from build123d import *

# Parameters (mm, degrees)
F0_W      = 57
F0_H      = 57
F1_DEPTH  = 49
F2_R      = 2
F3_R      = 2.55
F4_DEPTH  = 49.001
F5_R      = 2.55
F6_DEPTH  = 44
F7_R      = 3
F8_R      = 10
F9_DEPTH  = 2
F10_R     = 4
F11_DEPTH = 25
F12_R     = 19
F12_R_2   = 10
F13_DEPTH = 1.5


with BuildPart() as f1:
    # F0 (on Top) → F1 (new body)
    with BuildSketch(Plane.XY):
        Rectangle(F0_W, F0_H)
    extrude(amount=F1_DEPTH)

    # F2
    f2_edges = [f1.edges().sort_by_distance(p)[0] for p in [
        (-28.5, -28.5, 24.5),
        (28.5, -28.5, 24.5),
        (28.5, 28.5, 24.5),
        (-28.5, 28.5, 24.5),
    ]]
    fillet(f2_edges, radius=F2_R)

    # F3 (on face) → F4 (cut, through all)
    with BuildSketch(Plane(origin=(0, 0, 0), x_dir=(1, 0, 0), z_dir=(0, 0, -1))):
        with Locations((-23.5, -23.5)):
            Circle(F3_R)
        with Locations((-23.5, 23.5)):
            Circle(F3_R)
        with Locations((23.5, 23.5)):
            Circle(F3_R)
        with Locations((23.5, -23.5)):
            Circle(F3_R)
    extrude(amount=-F4_DEPTH, mode=Mode.SUBTRACT)

    # F5 (on face) → F6 (cut)
    with BuildSketch(Plane(origin=(0, 0, 0), x_dir=(1, 0, 0), z_dir=(0, 0, -1))):
        with BuildLine():
            Line((-26.5, -28.5), (-18.5, -28.5))
            Line((-18.5, -28.5), (-18.5, -18.5))
            Line((-18.5, -18.5), (-28.5, -18.5))
            Line((-28.5, -18.5), (-28.5, -26.5))
            ThreePointArc((-28.5, -26.5), (-27.9142135624, -27.9142135624), (-26.5, -28.5))
        make_face()
        with Locations((-23.5, -23.5)):
            Circle(F5_R, mode=Mode.SUBTRACT)
        with BuildLine():
            Line((28.5, -26.5), (28.5, -18.5))
            Line((28.5, -18.5), (18.5, -18.5))
            Line((18.5, -18.5), (18.5, -28.5))
            Line((18.5, -28.5), (26.5, -28.5))
            ThreePointArc((26.5, -28.5), (27.9142135624, -27.9142135624), (28.5, -26.5))
        make_face()
        with Locations((23.5, -23.5)):
            Circle(F5_R, mode=Mode.SUBTRACT)
        with BuildLine():
            Line((18.5, 18.5), (28.5, 18.5))
            Line((28.5, 18.5), (28.5, 26.5))
            ThreePointArc((28.5, 26.5), (27.9142135624, 27.9142135624), (26.5, 28.5))
            Line((26.5, 28.5), (18.5, 28.5))
            Line((18.5, 28.5), (18.5, 18.5))
        make_face()
        with Locations((23.5, 23.5)):
            Circle(F5_R, mode=Mode.SUBTRACT)
        with BuildLine():
            Line((-18.5, 18.5), (-18.5, 28.5))
            Line((-18.5, 28.5), (-26.5, 28.5))
            ThreePointArc((-26.5, 28.5), (-27.9142135624, 27.9142135624), (-28.5, 26.5))
            Line((-28.5, 26.5), (-28.5, 18.5))
            Line((-28.5, 18.5), (-18.5, 18.5))
        make_face()
        with Locations((-23.5, 23.5)):
            Circle(F5_R, mode=Mode.SUBTRACT)
    extrude(amount=-F6_DEPTH, mode=Mode.SUBTRACT)

    # F7
    f7_edges = [f1.edges().sort_by_distance(p)[0] for p in [
        (-18.5, -18.5, 22),
        (-18.5, -28.5, 22),
        (-28.5, -18.5, 22),
        (-28.5, 18.5, 22),
        (-18.5, 28.5, 22),
        (18.5, -28.5, 22),
        (28.5, -18.5, 22),
        (-18.5, 18.5, 22),
        (28.5, 18.5, 22),
        (18.5, 28.5, 22),
        (18.5, 18.5, 22),
        (18.5, -18.5, 22),
    ]]
    fillet(f7_edges, radius=F7_R)

    # F8 (on face) → F9 (cut)
    with BuildSketch(Plane.XY.offset(49)):
        Circle(F8_R)
    extrude(amount=-F9_DEPTH, mode=Mode.SUBTRACT)

    # F10 (on face) → F11 (cut)
    with BuildSketch(Plane.XY.offset(47)):
        Circle(F10_R)
    extrude(amount=-F11_DEPTH, mode=Mode.SUBTRACT)

    # F12 (on face) → F13 (join)
    with BuildSketch(Plane.XY.offset(49)):
        Circle(F12_R)
        Circle(F12_R_2, mode=Mode.SUBTRACT)
    extrude(amount=F13_DEPTH)


solid = f1.part
Read the model definition and answer for the solid it produces. Units are mm, in the model's axes. A direction names the side the tool comes from. Coordinates: 2 decimals unless noted, no trailing zeros. Order: outer loops, then holes, each group sorted by start corner. A loop starts at its lowest first (then second) coordinate and runs counter-clockwise, first axis right, second up. Notation, with made-up numbers: M 35.25,53.5 L 75.25,53.5 A32 cw 75.25,89.5 Z; hole C 42,31.5 d3. An arc over 180 degrees is marked long. Put each result on its own line as item: value. Start each with the question number.
Item 1: For faces 4 (the face through (27.64, -17.6, 22.31)), 5 (the face through (-23.54, 26.24, 44)), 6 (the face through (8, -8, 50.5)), 7 (the face through (24, 18.5, 22)), 8 (the face through (-23.5, -26.4, 44)), determine the directions among +Z, -Z, +X, -X, +Y, -Y from which every point of the face is accessible in a straight line to the end or side of a thin tool.
Item 2: Section A-A, the plane y = -23.5 is taken. Determine the outline of the cut face in (x, z), plus the area to 3 significant figures.
Item 3: Section B-B, the plane z = 30.5 is taken. Determine the outline of the cut face in (x, y).
Item 4: The mould has two halves that part along Y. Classify faces 1 (the face through (-25.4, -25.2, 46.5)), 2 (the face through (26.2, 23.4, 44)), 3 (the face through (27.93, 27.9, 46.54)): +Y half, -Y half, draft (parallel to the pull), parting line (faces both ways), or undercut.
Item 5: Section D-D, the plane y = 0 is taken. Determine the outline of the cut face in (x, z), plus the area to 3 significant figures.
Item 6: Consider probe 1 along X at (y, z) = (23.5, 46.95); probe 2 along Z at (x, y) = (4, 0.5). Determine where each line is inside the solid, lowest interval first. Write a range as [from, to].
Item 7: Given pin 1 Ø2 at (x, z) = (24.5, 31.5) entering from +Y; pin 2 Ø6 at (x, y) = (-9.5, 3) entering from -Z; pin 3 Ø2.5 at (x, y) = (0.5, -1.5) entering from +Z; pin 4 Ø4.5 at (x, z) = (24, 14.5) entering from -Y, each flat-ended and moving along its own axis, determine where each tip first touches the part or whether it passes through.
Computed:
1. face 4: -Z, +X, -Y
1. face 5: -Z, -X, +Y
1. face 6: +Z, +X, -X, +Y, -Y
1. face 7: -Z, +X, +Y
1. face 8: -Z, -X, -Y
2. outline: M -28.5,44 L -26.05,44 L -26.05,49 L -28.5,49 Z; M -20.95,44 L -18.5,44 L -18.5,0 L 18.5,0 L 18.5,44 L 20.95,44 L 20.95,49 L -20.95,49 Z; M 26.05,44 L 28.5,44 L 28.5,49 L 26.05,49 Z
2. area: 1,860 mm2
3. outline: M -28.5,-15.5 A3 ccw -25.5,-18.5 L -21.5,-18.5 A3 cw -18.5,-21.5 L -18.5,-25.5 A3 ccw -15.5,-28.5 L 15.5,-28.5 A3 ccw 18.5,-25.5 L 18.5,-21.5 A3 cw 21.5,-18.5 L 25.5,-18.5 A3 ccw 28.5,-15.5 L 28.5,15.5 A3 ccw 25.5,18.5 L 21.5,18.5 A3 cw 18.5,21.5 L 18.5,25.5 A3 ccw 15.5,28.5 L -15.5,28.5 A3 ccw -18.5,25.5 L -18.5,21.5 A3 cw -21.5,18.5 L -25.5,18.5 A3 ccw -28.5,15.5 Z; hole C 0,0 d8
4. face 1: undercut
4. face 2: draft
4. face 3: +Y half
5. outline: M -28.5,0 L 28.5,0 L 28.5,49 L 19,49 L 19,50.5 L 10,50.5 L 10,47 L 4,47 L 4,22 L -4,22 L -4,47 L -10,47 L -10,50.5 L -19,50.5 L -19,49 L -28.5,49 Z
5. area: 2,580 mm2
6. probe 1: x = [-28.5, -26.05], [-20.95, 20.95], [26.05, 28.5]
6. probe 2: z = [0, 47]
7. pin 1: stops at y = 18.5
7. pin 2: stops at z = 0
7. pin 3: stops at z = 22
7. pin 4: stops at y = -18.5
